from build123d import *

# Parameters (mm, degrees)
SKETCH1_W           = 15
SKETCH1_H           = 20
BOSS_EXTRUDE1_DEPTH = 1
SKETCH2_W           = 9.75
SKETCH2_H           = 12
BOSS_EXTRUDE2_DEPTH = 2


with BuildPart() as part:
    # Sketch1 → Boss-Extrude1 (new body)
    with BuildSketch(Plane.XY):
        Rectangle(SKETCH1_W, SKETCH1_H)
    extrude(amount=-BOSS_EXTRUDE1_DEPTH)

    # Sketch2 → Boss-Extrude2 (add)
    with BuildSketch(Plane.XY):
        Rectangle(SKETCH2_W, SKETCH2_H)
    extrude(amount=-BOSS_EXTRUDE2_DEPTH)


solid = part.part
The model under review builds one solid part; all positions refer to its coordinate system, in mm. A direction names the side the tool comes from. Round coordinates to 2 decimals unless told otherwise and drop trailing zeros. Loops run counter-clockwise (first coordinate to the right, second up) from the corner with the lowest first, then second, coordinate; pieces in that order, holes last. Notation, with made-up numbers: (29.25, 65) -> (69.25, 65) arc R35 ccw to (69.25, 101) -> close; hole circle Ø8 at (38, 43). An arc over 180 degrees is marked (long way). One line per question, with ' | ' between items. Start each with the question number.
Item 1: For pin 1 (1 mm diameter, centred on x = 6, y = 6, fed in from -Z); pin 2 (0.8 mm diameter, centred on x = 0.5, z = -1.5, fed in from -Y); pin 3 (5 mm diameter, centred on x = 1.5, y = 7, fed in from -Z); pin 4 (0.5 mm diameter, centred on y = 0, z = -1.5, fed in from -X) (3 decimals), all flat-tipped, find the tip position at first contact; note any pin that passes through.
Item 2: Wall thickness on line 1 along Y through (x, z) = (4, -1.5); line 2 along Z through (x, y) = (4.75, 9.25); line 3 along X through (y, z) = (-4, -1.5) (3 decimals): over which ranges is each line inside the solid? List them lowest first. Write a range as [from, to].
Item 3: Add section B-B, the plane x = 0. Write out the cut boundary in (y, z), then the cut area to 3 significant figures.
Item 4: Add section A-A, the plane y = 3. Write out the cut boundary in (x, z) (3 decimals).
Item 5: Add section C-C, the plane z = -1.6. Write out the cut boundary in (x, y) (3 decimals).
Item 6: Add section D-D, the plane x = 5.5. Write out the cut boundary in (y, z), then the cut area to 3 significant figures.
Item 7: Machinability: for faces 1 (the face through (-0.1, 6, -1.5)), 2 (the face through (-4.875, -0.1, -1.5)), 3 (the face through (4.875, -0.1, -1.5)), which of the approach directions +Z, -Z, +X, -X, +Y, -Y give a long, thin tool a straight path to every point of the face, cutting with its end or side? Answer none if there is none.
Return value:
1) pin 1: stops at z = -1 | pin 2: stops at y = -6 | pin 3: stops at z = -2 | pin 4: stops at x = -4.875
2) line 1: y = [-6, 6] | line 2: z = [-1, 0] | line 3: x = [-4.875, 4.875]
3) outline: (-10, -1) -> (-6, -1) -> (-6, -2) -> (6, -2) -> (6, -1) -> (10, -1) -> (10, 0) -> (-10, 0) -> close | area: 32.0 mm2
4) outline: (-7.5, -1) -> (-4.875, -1) -> (-4.875, -2) -> (4.875, -2) -> (4.875, -1) -> (7.5, -1) -> (7.5, 0) -> (-7.5, 0) -> close
5) outline: (-4.875, -6) -> (4.875, -6) -> (4.875, 6) -> (-4.875, 6) -> close
6) outline: (-10, -1) -> (10, -1) -> (10, 0) -> (-10, 0) -> close | area: 20.0 mm2
7) face 1: -Z, +X, -X, +Y | face 2: -Z, -X, +Y, -Y | face 3: -Z, +X, +Y, -Y
